from build123d import *

# Parameters (mm, degrees)
SKETCH1_W                = 20
SKETCH1_H                = 132.062590847
SKETCH1_W_2              = 173.191489362
SKETCH1_H_2              = 20
BOSS_EXTRUDE1_DEPTH      = 40
BOSS_EXTRUDE2_DEPTH      = 200
BOSS_EXTRUDE2_DEPTH_BACK = 160


with BuildPart() as part:
    # Sketch1 → Boss-Extrude1 (new body)
    with BuildSketch(Plane(origin=(0, 0, 0), x_dir=(1, 0, 0), z_dir=(0, 1, 0))):
        with Locations((10, 86.031295423)):
            Rectangle(SKETCH1_W, SKETCH1_H)
        Polygon((20, 60), (20, 20), (20, 0), (24, 0), (24, 60), align=None)
        Polygon((20, -20), (0, -20), (0, 0), (0, 20), (20, 20), align=None)
        with Locations((-86.595744681, -10)):
            Rectangle(SKETCH1_W_2, SKETCH1_H_2)
        Polygon((20, -20), (0, -20), (-40, -20), (-40, -24), (20, -24), align=None)
    extrude(amount=BOSS_EXTRUDE1_DEPTH)

    # Sketch1_3 → Boss-Extrude2 (add, two sides)
    with BuildSketch(Plane(origin=(0, 0, 0), x_dir=(1, 0, 0), z_dir=(0, 1, 0))) as boss_extrude2_sk:
        Polygon((20, -20), (0, -20), (0, 0), (0, 20), (20, 20), align=None)
    extrude(amount=BOSS_EXTRUDE2_DEPTH)
    extrude(boss_extrude2_sk.sketch, amount=-BOSS_EXTRUDE2_DEPTH_BACK)


solid = part.part
For this review, take the finished solid that the model builds, in its own axes (mm). A direction names the side the tool comes from. Round coordinates to 2 decimals unless told otherwise and drop trailing zeros. Order: outer loops, then holes, each group sorted by start corner. A loop starts at its lowest first (then second) coordinate and runs counter-clockwise, first axis right, second up. Notation, with made-up numbers: (-29.75, -21.75) -> (22.25, -21.75) arc R15 ccw to (22.25, -8.75) -> close; hole circle Ø2 at (0.5, 33). An arc over 180 degrees is marked (long way). Put each result on its own line as item: value.
Q1. Insertion check: pin 1 Ø4 at (y, z) = (40.5, -76) entering from +X; pin 2 Ø20 at (x, y) = (-114, 16.5) entering from +Z; pin 3 Ø7 at (x, z) = (15, -89) entering from +Y. Each pin has a flat end and moves straight along its axis. Give the tip position at first contact, or say it passes through.
Check result:
pin 1: x = 20
pin 2: z = 20
pin 3: y = 40
Q2. Add section A-A on y = 12. Write out the cut boundary in (x, z).
Check result:
outline: (-173.19, 0) -> (0, 0) -> (0, -152.06) -> (20, -152.06) -> (20, -60) -> (24, -60) -> (24, 0) -> (20, 0) -> (20, 24) -> (-40, 24) -> (-40, 20) -> (-173.19, 20) -> close
Q3. Add section B-B on z = 5. Write out the cut boundary in (x, y).
Check result:
outline: (-173.19, 0) -> (0, 0) -> (0, -160) -> (20, -160) -> (20, 200) -> (0, 200) -> (0, 40) -> (-173.19, 40) -> close
Q4. Add section D-D on y = 158.5. Write out the cut boundary in (x, z).
Check result:
outline: (0, -20) -> (20, -20) -> (20, 20) -> (0, 20) -> close
Q5. Machinability: for faces 1 (the flat face through (10, -79, 20)), 2 (the flat face through (-108, 20, 20)), 3 (the flat face through (10, 119, -20)), which of the approach directions +Z, -Z, +X, -X, +Y, -Y give a long, thin tool a straight path to every point of the face, cutting with its end or side? Answer none if there is none.
Check result:
face 1: +Z, +X, -X, -Y
face 2: +Z, -X, +Y, -Y
face 3: -Z, +X, -X, +Y
Q6. Add section C-C on x = -145.5. Write out the cut boundary in (y, z).
Check result:
outline: (0, 0) -> (40, 0) -> (40, 20) -> (0, 20) -> close
Q7. For probe 1 along Z at (x, y) = (-49, 35); probe 2 along X at (y, z) = (38, -5), list the stretches that pass through material, from the lowest coordinate up. Write a range as [from, to].
Check result:
probe 1: [0, 20]
probe 2: [0, 24]
